```python
from build123d import *

# Parameters (mm, degrees)
ESQUISSE3_R                  = 1.25
BOSS_EXTRU_1_DEPTH           = 12.5
R_P_TITION_CIRCULAIRE1_COUNT = 3
ESQUISSE2_R                  = 1
ENL_V_MAT_EXTRU_2_DEPTH      = 7.0000001


with BuildPart() as part:
    # Esquisse1 → Base-Révolution (revolve)
    with BuildSketch(Plane.XY):
        with BuildLine():
            Line((0, 3), (4.039392014, 3))
            ThreePointArc((4.039392014, 3), (4.5, 0), (4.039392014, -3))
            Line((4.039392014, -3), (0, -3))
            Line((0, -3), (0, 3))
        make_face()
    revolve(axis=Axis((0, -3, 0), (0, 1, 0)))

    # Esquisse3 → Boss.-Extru.1 (add)
    with BuildSketch(Plane.XY):
        Circle(ESQUISSE3_R)
    boss_extru_1 = extrude(amount=BOSS_EXTRU_1_DEPTH)

    # Répétition circulaire1: Boss.-Extru.1 ×3 about axis
    r_p_tition_circulaire1_axis = Axis((0, -3, 0), (0, 1, 0))
    for i in range(1, R_P_TITION_CIRCULAIRE1_COUNT):
        add(boss_extru_1.rotate(r_p_tition_circulaire1_axis, i * 360 / R_P_TITION_CIRCULAIRE1_COUNT))

    # Esquisse2 → Enlèv. mat.-Extru.2 (cut, through all)
    with BuildSketch(Plane.XZ.offset(3)):
        Circle(ESQUISSE2_R)
    extrude(amount=-ENL_V_MAT_EXTRU_2_DEPTH, mode=Mode.SUBTRACT)


solid = part.part
```
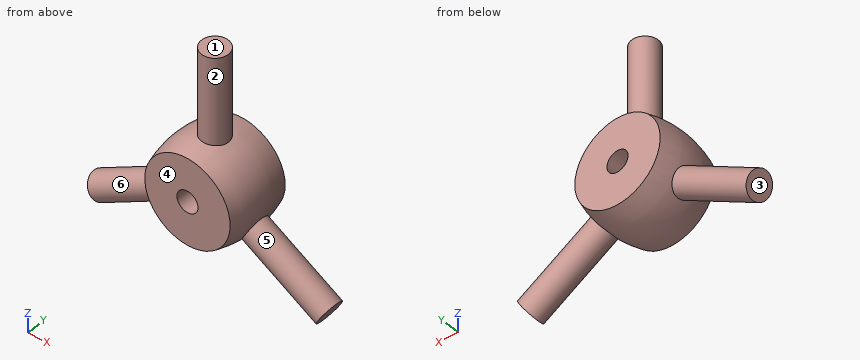
The listing builds one solid part. Answer for the finished solid, in the listing's coordinates (mm). Face numbers are marked on the shaded views. A direction names the side the tool comes from. Give positions to 0.01 mm unless a question says otherwise; leave off trailing zeros. Order: outer loops, then holes, each group sorted by start corner. A loop starts at its lowest first (then second) coordinate and runs counter-clockwise, first axis right, second up. Notation, with made-up numbers: (61.5, -26.75) -> (101.5, -26.75) arc R17 cw to (101.5, 4.25) -> close; hole circle Ø6 at (-22.75, 24.25). An arc over 180 degrees is marked (long way). One line per item, written item: value.
1) Determine the mould class of the marked faces 3, 4, 5 and 6 for opening direction X: pulls with the +X half, pulls with the -X half, needs draft (parallel to the pull), parting line crosses it, or undercut.
Reported:
face 3: pulls with the -X half
face 4: needs draft
face 5: undercut
face 6: undercut
2) A flat-ended cylindrical pin translates along its axis: P1, Ø8, axis at x = 9, z = 3, coming from the +Y side. Find the tip coordinate at first contact, or state that the pin passes through.
Reported:
P1: passes through
3) A tool of negligible diameter and unlimited length cuts with its end or side. For the marked faces 1 and 2, from which of +Z, -Z, +X, -X, +Y, -Y can it reach the whole face along a straight path? Write none if from no direction.
Reported:
face 1: +Z, +X, -X, +Y, -Y
face 2: +Z
4) Find section A-A, the plane z = 5. Determine the outline of the cut face in (x, y).
Reported:
outline: circle Ø2.5 at (0, 0)
5) Find the intervals of material crossed by line 1 (X direction, y = -0.75, z = 5.25); line 2 (Z direction, x = 0, y = -0.8), in increasing order.
Reported:
line 1: x = -1 to 1
line 2: z = -4.47 to -1, 1 to 12.5
